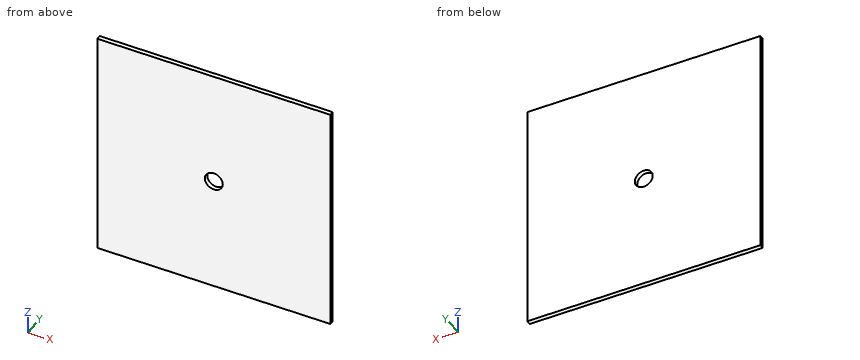
from build123d import *

# Parameters (mm, degrees)
SKETCH1_W       = 13
SKETCH1_H       = 13
MESH_DEPTH      = 0.25
SKETCH2_R       = 0.5
HOLE_DEPTH      = 10
HOLE_DEPTH_BACK = 10


with BuildPart() as part:
    # Sketch1 → Mesh (new body)
    with BuildSketch(Plane(origin=(0, 0, 0), x_dir=(1, 0, 0), z_dir=(0, 1, 0))):
        Rectangle(SKETCH1_W, SKETCH1_H)
    extrude(amount=MESH_DEPTH)

    # Sketch2 → Hole (cut, two sides)
    with BuildSketch(Plane(origin=(0, 0.25, 0), x_dir=(1, 0, 0), z_dir=(0, 1, 0))) as hole_sk:
        Circle(SKETCH2_R)
    extrude(amount=HOLE_DEPTH, mode=Mode.SUBTRACT)
    extrude(hole_sk.sketch, amount=-HOLE_DEPTH_BACK, mode=Mode.SUBTRACT)


solid = part.part
The model under review builds one solid part; all positions refer to its coordinate system, in mm. Round coordinates to 2 decimals unless told otherwise and drop trailing zeros. Order: outer loops, then holes, each group sorted by start corner. A loop starts at its lowest first (then second) coordinate and runs counter-clockwise, first axis right, second up. Notation, with made-up numbers: (-10.75, 66.5) -> (43.25, 66.5) arc R29 cw to (43.25, 99.5) -> close; hole circle Ø11 at (-8, 59). An arc over 180 degrees is marked (long way). Return JSON: item names as keys, results as strings.
1. Take a section at B-B (x = 0). Write out the cut boundary in (y, z), then the cut area to 3 significant figures.
Answer block:
{"outline": "(0, -6.5) -> (0.25, -6.5) -> (0.25, -0.5) -> (0, -0.5) -> close; (0, 0.5) -> (0.25, 0.5) -> (0.25, 6.5) -> (0, 6.5) -> close", "area": "3.00 mm²"}
2. Take a section at A-A (z = 0). Write out the cut boundary in (x, y), then the cut area to 3 significant figures.
Answer block:
{"outline": "(-6.5, 0) -> (-0.5, 0) -> (-0.5, 0.25) -> (-6.5, 0.25) -> close; (0.5, 0) -> (6.5, 0) -> (6.5, 0.25) -> (0.5, 0.25) -> close", "area": "3.00 mm²"}
3. For L1, parallel to Z at x = 0, y = 0.1; L2, parallel to X at y = 0.15, z = -0.25, list the stretches that pass through material, from the lowest coordinate up. Write a range as [from, to].
Answer block:
{"L1": "z = [-6.5, -0.5], [0.5, 6.5]", "L2": "x = [-6.5, -0.43], [0.43, 6.5]"}
4. Insertion check: P1, Ø4, axis at x = 3.5, z = -2, coming from the -Y side. The pin has a flat end and moves straight along its axis. Give the tip position at first contact, or say it passes through.
Answer block:
{"P1": "stops at y = 0"}
